Build history of the part. All positions in model axes, mm. Face numbers are marked on the shaded views. A direction names the side the tool comes from. Give positions to 0.01 mm unless a question says otherwise; leave off trailing zeros. Loops run counter-clockwise (first coordinate to the right, second up) from the corner with the lowest first, then second, coordinate; pieces in that order, holes last. Notation, with made-up numbers: M 77,26 L 120,26 A17 cw 120,33 Z; hole C 10.5,68 d10. An arc over 180 degrees is marked long. Put each result on its own line as item: value.
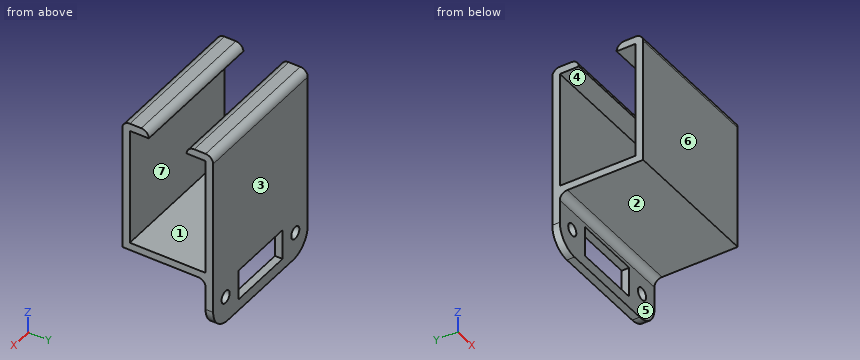
Autodesk Fusion 360 part; units mm, degrees
sketch "Sketch1" plane through (0, 0, 0) normal (1, 0, 0) x (0, 0, -1)
  line L0 (0, 0) -> (-14, 0)
  line L1 (-14, 0) -> (-14, 2)
  line L2 (-14, 2) -> (0, 2)
  line L3 (0, 2) -> (0, 0)
  dimension "d1" = 14
  dimension "d2" = 2
extrude "Extrude1" add sketch "Sketch1" along normal blind 38
fillet "Fillet1" radius 5.9 4 edges at (0, 1, 14) (38, 1, 14) (38, 1, 0) (0, 1, 0)
sketch "Sketch2" plane through (0, 2, 0) normal (0, 1, 0) x (-1, 0, 0)
  arc A0 (-5.9, 0) -> (0, 5.9) centre (-5.9, 5.9) ccw
  line L0 (0, 5.9) -> (0, 8.1)
  arc A1 (0, 8.1) -> (-5.9, 14) centre (-5.9, 8.1) ccw
  line L1 (-5.9, 14) -> (-32.1, 14)
  arc A2 (-32.1, 14) -> (-38, 8.1) centre (-32.1, 8.1) ccw
  line L2 (-38, 8.1) -> (-38, 5.9)
  arc A3 (-38, 5.9) -> (-32.1, 0) centre (-32.1, 5.9) ccw
  line L3 (-32.1, 0) -> (-5.9, 0)
  line L4 (-19, 0) -> (-19, 14)
  line L5 (-19, 7) -> (-27.875, 7)
  line L6 (-27.875, 7) -> (-27.875, 3)
  line L7 (-27.875, 3) -> (-19, 3)
  line L8 (-19, 3) -> (-19, 7)
  line L9 (-27.875, 3) -> (-10.125, 3)
  line L10 (-10.125, 3) -> (-10.125, 11)
  line L11 (-10.125, 11) -> (-27.875, 11)
  line L12 (-27.875, 11) -> (-27.875, 3)
  line L13 (-10.125, 7) -> (-6.625, 7)
  circle A4 centre (-5, 7) radius 1.625
  line L14 (-27.875, 7) -> (-31.375, 7)
  circle A5 centre (-33, 7) radius 1.625
  dimension "d7" = 8.875
  dimension "d8" = 4
  dimension "d9" = 17.75
  dimension "d10" = 8
  dimension "d11" = 3.5
  dimension "d12" = 3.25
  dimension "d13" = 3.5
  dimension "d14" = 3.25
extrude "Extrude2" cut sketch "Sketch2" against normal blind 2 contours A4 | A5 | L4 L5 L6 L7 L8 L9 L12 | L4 L8 L9 L10 L11 | L4 L5 L11 L12
sketch "Sketch3" plane through (0, 2, 0) normal (0, 1, 0) x (-1, 0, 0)
  circle A0 centre (-33, 7) radius 1.625
  circle A1 centre (-5, 7) radius 1.625
  line L0 (-10.125, 3) -> (-27.875, 3)
  line L1 (-27.875, 3) -> (-27.875, 11)
  line L2 (-27.875, 11) -> (-10.125, 11)
  line L3 (-10.125, 11) -> (-10.125, 3)
  arc A2 (-5.9, 0) -> (0, 5.9) centre (-5.9, 5.9) ccw
  line L4 (0, 5.9) -> (0, 8.1)
  arc A3 (0, 8.1) -> (-5.9, 14) centre (-5.9, 8.1) ccw
  line L5 (-5.9, 14) -> (-32.1, 14)
  arc A4 (-32.1, 14) -> (-38, 8.1) centre (-32.1, 8.1) ccw
  line L6 (-38, 8.1) -> (-38, 5.9)
  arc A5 (-38, 5.9) -> (-32.1, 0) centre (-32.1, 5.9) ccw
  line L7 (-32.1, 0) -> (-5.9, 0)
  line L8 (-32.1, 14) -> (-32.1, 45)
  line L9 (-32.1, 45) -> (-38, 45)
  line L10 (-38, 45) -> (-38, 8.1)
  line L11 (-38, 8.1) -> (-32.1, 8.1)
  line L12 (-32.1, 8.1) -> (-32.1, 45)
  line L13 (-38, 45) -> (0, 45)
  line L14 (0, 45) -> (0, 8.1)
  line L15 (0, 8.1) -> (-38, 8.1)
  line L16 (-38, 8.1) -> (-38, 45)
  dimension "d17" = 31
extrude "Extrude3" add sketch "Sketch3" against normal blind 2 contours A4 L8 L9 L10 L12 L13 L16 | A3 L5 L8 L12 L13 L14
sketch "Sketch4" plane through (38, 0, 0) normal (1, 0, 0) x (0, 0, -1)
  line L0 (-5.9, 0) -> (-5.9, 2)
  line L1 (-5.9, 2) -> (-45, 2)
  line L2 (-45, 2) -> (-45, 0)
  line L3 (-45, 0) -> (-5.9, 0)
  line L4 (-45, 0) -> (-45, -5)
  line L5 (-45, -5) -> (-47, -5)
  line L6 (-47, -5) -> (-45, -5)
  line L7 (-45, -5) -> (-45, 2)
  line L8 (-45, 2) -> (-47, 2)
  line L9 (-47, 2) -> (-47, -5)
  line L10 (-45, 0) -> (-14, 0)
  line L11 (-14, 0) -> (-14, -20)
  line L12 (-14, -20) -> (-45, -20)
  line L13 (-45, -20) -> (-45, -15)
  line L14 (-45, -15) -> (-47, -15)
  line L15 (-47, -15) -> (-47, -22)
  line L16 (-47, -22) -> (-14, -22)
  line L17 (-14, -22) -> (-12, -22)
  line L18 (-12, -22) -> (-12, 0)
  line L19 (-12, 0) -> (-14, 0)
  line L20 (-14, 0) -> (-14, -22)
  dimension "d20" = 5
  dimension "d21" = 2
  dimension "d22" = 31
  dimension "d23" = 20
  dimension "d24" = 31
  dimension "d25" = 5
  dimension "d26" = 2
  dimension "d27" = 7
  dimension "d28" = 33
  dimension "d29" = 2
  dimension "d30" = 22
extrude "Extrude4" add sketch "Sketch4" against normal blind 38 contours L3 L11 L17 L18 L19 L20 | L2 L4 L5 L6 L7 L8 L9 | L12 L13 L14 L15 L16 L20
move_face "MoveFace1" by (0, 0, 2) 6 faces at (25.3333, -14.6667, 12) (25.3333, -6.6667, 14) (25.3333, -17.3333, 47) (25.3333, -18.3333, 45) (25.3333, -1.6667, 45) (25.3333, -0.3333, 47)
fillet "Fillet2" radius 2 1 edges at (19, 0, 14)
fillet "Fillet3" radius 2 1 edges at (19, 2, 49)
fillet "Fillet4" radius 2 1 edges at (19, -22, 49)
fillet "Fillet5" radius 2 2 edges at (19, -5, 49) (19, -15, 49)
equation "d7 = ( 17.75 / 2 ) * 1 mm"
equation "d9 = 8.875 mm * 2"
equation "d10 = 4.000 mm * 2"
Q1. Probe line 1 (Z direction, x = 28, y = -17.5); line 2 (Y direction, x = 22, z = 34); line 3 (Y direction, x = 29.5, z = 9.5). List the from-to ranges inside material, lowest first. Write a range as from..to.
Here are the results:
line 1: 14..16, 47..49
line 2: -22..-20, 0..2
line 3: 0..2
Q2. Tool access for the marked faces 5, 6 and 7: list every direction of +Z, -Z, +X, -X, +Y, -Y with a clear straight run to the whole face (end or side of a thin tool).
Here are the results:
face 5: -Z, +X, -X, -Y
face 6: +Z, -Z, +X, -X, -Y
face 7: +X, -X
Q3. Slice it at C-C (z = 7). List the corners of the cut face in (x, y) (3 decimals).
Here are the results:
outline: M 0,0 L 3.375,0 L 3.375,2 L 0,2 Z; M 6.625,0 L 10.125,0 L 10.125,2 L 6.625,2 Z; M 27.875,0 L 31.375,0 L 31.375,2 L 27.875,2 Z; M 34.625,0 L 38,0 L 38,2 L 34.625,2 Z
Q4. Drop flat-ended pins along their axis: pin 1 Ø3 at (x, z) = (5, 7) entering from -Y; pin 2 Ø5 at (x, z) = (33, 7) entering from -Y; pin 3 Ø1.5 at (x, y) = (22, -3) entering from -Z; pin 4 Ø0.6 at (x, y) = (15.5, 1.5) entering from +Z. Give the stop position or say it passes through.
Here are the results:
pin 1: through
pin 2: y = 0
pin 3: z = 14
pin 4: z = 48.6
Q5. Mould opens along Y. For the marked faces 1, 2, 3 and 4 say: pulls with the +Y half, pulls with the -Y half, needs draft (parallel to the pull), parting line crosses it, or undercut.
Here are the results:
face 1: undercut
face 2: needs draft
face 3: pulls with the +Y half
face 4: undercut
Q6. Slice it at B-B (z = 26.5). List the corners of the cut face in (x, y), and give its area (3 significant figures).
Here are the results:
outline: M 0,-22 L 38,-22 L 38,-20 L 0,-20 Z; M 0,0 L 38,0 L 38,2 L 0,2 Z
area: 152 mm²
